Here's how the part is built. I have some questions about the finished solid (model axes, mm). A direction names the side the tool comes from. Coordinates: 2 decimals unless noted, no trailing zeros. Write each loop counter-clockwise with the first axis right and the second up, starting at its lowest first coordinate (ties: lowest second). Pieces come first, ordered by that corner, then holes.
Item 1: If we section it at C-C (x = 7): Count the separate pieces of the cut face and the enclosed holes in it, then the cut area to 3 significant figures.
Item 2: For faces 4 (the face through (-27.75, 4.08, 36.34)), 5 (the face through (-28.414, 5.42, 32.282)), 6 (the face through (23, 5, 31)), 7 (the face through (0, 30, 1)), 8 (the face through (20, 13, 36)), which set-ups out of +Z, -Z, +X, -X, +Y, -Y let a thin tool reach every point of the face, with its end or its side?
Item 3: I'm going to push flat-ended pins straight in: pin 1 Ø0.8 at (x, z) = (-26, 32.5) entering from -Y; pin 2 Ø2 at (y, z) = (9.5, -29.5) entering from -X; pin 3 Ø4.5 at (x, y) = (-24.5, 4.5) entering from -Z; pin 4 Ø1.7 at (x, y) = (27, 4) entering from -Z. Where does each tip first touch, or does it pass through?
Item 4: If I drill on line 1 (Y direction, x = 26, z = 35); line 2 (X direction, y = 4, z = 29); line 3 (X direction, y = 8.1, z = 29), over which ranges is the centre line in solid material (lowest first)?
Item 5: If we section it at D-D (x = 16.5): Please give me the cut outline in (y, z).
Item 6: If we section it at A-A (z = 29): Please give me the cut outline in (x, y).
Item 7: If we section it at B-B (y = 20): Please give me the cut outline in (x, z), then the cut area to 3 significant figures.
Item 8: We'd pull the mould along Z, two halves only. Please class faces 1 (the face through (30, 29, 35)), 2 (the face through (9, 5.9, 31)), 3 (the face through (0, 13, -39)): +Z half, -Z half, draft (parallel to the pull), parting line (faces both ways), or undercut.
from build123d import *

# Parameters (mm, degrees)
SKETCH_1_W                 = 44
SKETCH_1_H                 = 78
EXTRUDE_1_DEPTH            = 33
SHELL_1_T                  = -3
SHELL_1_THICKNESS_2_FACE_W = 75
SHELL_1_THICKNESS_2_FACE_H = 38
SHELL_1_THICKNESS_2_DEPTH  = 7
SKETCH_3_R                 = 3.6
CUT_EXTRUDE_1_DEPTH        = 4.1
CUT_EXTRUDE_2_REACH        = 52.339
SKETCH_4_R                 = 2.25
SKETCH_5_W                 = 3
SKETCH_5_H                 = 3
CUT_EXTRUDE_3_DEPTH        = 6
SKETCH_6_W                 = 8
SKETCH_6_H                 = 8
SKETCH_6_R                 = 1.75
EXTRUDE_2_DEPTH            = 8
CUT_EXTRUDE_4_DEPTH        = 2.6
CUT_EXTRUDE_5_REACH        = 89.258
SKETCH_8_R                 = 5
CUT_EXTRUDE_6_REACH        = 61.245
SKETCH_9_R                 = 3.6


with BuildPart() as part:
    # 草圖1 → 填料-伸長1 (new body)
    with BuildSketch(Plane(origin=(0, 0, 0), x_dir=(1, 0, 0), z_dir=(0, 1, 0))):
        Rectangle(SKETCH_1_W, SKETCH_1_H)
    extrude(amount=EXTRUDE_1_DEPTH)

    # 薄殼1
    shell_1_openings = [part.faces().sort_by_distance(p)[0] for p in [
        (0, 16.5, 39),
    ]]
    offset(amount=SHELL_1_T, openings=shell_1_openings, kind=Kind.INTERSECTION)

    # 薄殼1 thickness 2 face (on inner face of the shell) → 薄殼1 thickness 2 (add)
    with BuildSketch(Plane(origin=(0, 3, 1.5), x_dir=(0, 0, -1), z_dir=(0, -1, 0))):
        Rectangle(SHELL_1_THICKNESS_2_FACE_W, SHELL_1_THICKNESS_2_FACE_H)
    extrude(amount=-SHELL_1_THICKNESS_2_DEPTH)

    # 草圖3 → 除料-伸長1 (cut)
    with BuildSketch(Plane(origin=(0, 10, 0), x_dir=(1, 0, 0), z_dir=(0, 1, 0))):
        with Locations(Location((7, 7, 0), (0, 0, 270))):
            Circle(SKETCH_3_R)
        with Locations(Location((7, -29, 0), (0, 0, 270))):
            Circle(SKETCH_3_R)
    extrude(amount=-CUT_EXTRUDE_1_DEPTH, mode=Mode.SUBTRACT)

    # 草圖4 → 除料-伸長2 (cut, up to next)
    with BuildSketch(Plane(origin=(0, 10, 0), x_dir=(1, 0, 0), z_dir=(0, 1, 0)), mode=Mode.PRIVATE) as cut_extrude_2_sk1:
        with Locations(Location((7, 7, 0), (0, 0, 270))):
            Circle(SKETCH_4_R)
    cut_extrude_2_tool1 = extrude(cut_extrude_2_sk1.sketch, amount=-CUT_EXTRUDE_2_REACH, mode=Mode.PRIVATE) & part.part
    # 草圖4 → 除料-伸長2 (cut, up to next)
    with BuildSketch(Plane(origin=(0, 10, 0), x_dir=(1, 0, 0), z_dir=(0, 1, 0)), mode=Mode.PRIVATE) as cut_extrude_2_sk2:
        with Locations(Location((7, -29, 0), (0, 0, 270))):
            Circle(SKETCH_4_R)
    cut_extrude_2_tool2 = extrude(cut_extrude_2_sk2.sketch, amount=-CUT_EXTRUDE_2_REACH, mode=Mode.PRIVATE) & part.part
    add(cut_extrude_2_tool1.solids().sort_by_distance((7, 10, -7))[0], mode=Mode.SUBTRACT)
    add(cut_extrude_2_tool2.solids().sort_by_distance((7, 10, 29))[0], mode=Mode.SUBTRACT)

    # 草圖5 → 除料-伸長3 (cut)
    with BuildSketch(Plane.XY.offset(39)):
        with Locations((20.5, 11.5)):
            Rectangle(SKETCH_5_W, SKETCH_5_H)
    extrude(amount=-CUT_EXTRUDE_3_DEPTH, mode=Mode.SUBTRACT)

    # 草圖6 → 填料-伸長2 (add)
    with BuildSketch(Plane.XY.offset(39)):
        with Locations((-26, 29)):
            Rectangle(SKETCH_6_W, SKETCH_6_H)
        with Locations((-26, 29)):
            Circle(SKETCH_6_R, mode=Mode.SUBTRACT)
        with Locations((-26, 4)):
            Rectangle(SKETCH_6_W, SKETCH_6_H)
        with Locations((-26, 4)):
            Circle(SKETCH_6_R, mode=Mode.SUBTRACT)
        with Locations((26, 4)):
            Rectangle(SKETCH_6_W, SKETCH_6_H)
        with Locations(Location((26, 4, 0), (0, 0, 180))):
            Circle(SKETCH_6_R, mode=Mode.SUBTRACT)
        with Locations((26, 29)):
            Rectangle(SKETCH_6_W, SKETCH_6_H)
        with Locations(Location((26, 29, 0), (0, 0, 180))):
            Circle(SKETCH_6_R, mode=Mode.SUBTRACT)
    extrude(amount=-EXTRUDE_2_DEPTH)

    # 草圖7 → 除料-伸長4 (cut)
    with BuildSketch(Plane(origin=(0, 0, 31), x_dir=(-1, 0, 0), z_dir=(0, 0, -1))):
        Polygon((27.616580754, 6.8), (29.233161507, 4), (27.616580754, 1.2), (24.383419246, 1.2), (22.766838493, 4), (24.383419246, 6.8), align=None)
        Polygon((-22.766838493, 29), (-24.383419246, 31.8), (-27.616580754, 31.8), (-29.233161507, 29), (-27.616580754, 26.2), (-24.383419246, 26.2), align=None)
        Polygon((-29.233161507, 4), (-27.616580754, 1.2), (-24.383419246, 1.2), (-22.766838493, 4), (-24.383419246, 6.8), (-27.616580754, 6.8), align=None)
        Polygon((24.383419246, 26.2), (22.766838493, 29), (24.383419246, 31.8), (27.616580754, 31.8), (29.233161507, 29), (27.616580754, 26.2), align=None)
    extrude(amount=-CUT_EXTRUDE_4_DEPTH, mode=Mode.SUBTRACT)

    # 草圖8 → 除料-伸長5 (cut, up to next)
    with BuildSketch(Plane.XY.offset(-36), mode=Mode.PRIVATE) as cut_extrude_5_sk1:
        with Locations((0, 20)):
            Circle(SKETCH_8_R)
    cut_extrude_5_tool1 = extrude(cut_extrude_5_sk1.sketch, amount=-CUT_EXTRUDE_5_REACH, mode=Mode.PRIVATE) & part.part
    add(cut_extrude_5_tool1.solids().sort_by_distance((0, 20, -36))[0], mode=Mode.SUBTRACT)

    # 草圖9 → 除料-伸長6 (cut, up to next)
    with BuildSketch(Plane(origin=(0, 33, 0), x_dir=(1, 0, 0), z_dir=(0, 1, 0)), mode=Mode.PRIVATE) as cut_extrude_6_sk1:
        with Locations(Location((7, 7, 0), (0, 0, 270))):
            Circle(SKETCH_9_R)
    cut_extrude_6_tool1 = extrude(cut_extrude_6_sk1.sketch, amount=-CUT_EXTRUDE_6_REACH, mode=Mode.PRIVATE) & part.part
    # 草圖9 → 除料-伸長6 (cut, up to next)
    with BuildSketch(Plane(origin=(0, 33, 0), x_dir=(1, 0, 0), z_dir=(0, 1, 0)), mode=Mode.PRIVATE) as cut_extrude_6_sk2:
        with Locations(Location((7, -29, 0), (0, 0, 270))):
            Circle(SKETCH_9_R)
    cut_extrude_6_tool2 = extrude(cut_extrude_6_sk2.sketch, amount=-CUT_EXTRUDE_6_REACH, mode=Mode.PRIVATE) & part.part
    add(cut_extrude_6_tool1.solids().sort_by_distance((7, 33, -7))[0], mode=Mode.SUBTRACT)
    add(cut_extrude_6_tool2.solids().sort_by_distance((7, 33, 29))[0], mode=Mode.SUBTRACT)


solid = part.part
Answer list:
1. separate pieces: 5
1. enclosed holes: 0
1. area: 919 mm2
2. face 4: +Z, -Z
2. face 5: -Z
2. face 6: -Z, +X, +Y, -Y
2. face 7: +Z
2. face 8: +Z, +X
3. pin 1: stops at y = 0
3. pin 2: stops at x = -22
3. pin 3: stops at z = 31
3. pin 4: stops at z = 33.6
4. line 1: y = 0 to 2.25, 5.75 to 8, 25 to 27.25, 30.75 to 33
4. line 2: x = -22 to 4.75, 9.25 to 22
4. line 3: x = -22 to 3.4, 10.6 to 22
5. outline: (0, -39) - (33, -39) - (33, 39) - (30, 39) - (30, -36) - (10, -36) - (10, 39) - (0, 39) - close
6. outline: (-22, 0) - (4.75, 0) - (4.75, 5.9) - (3.4, 5.9) - (3.4, 10) - (-19, 10) - (-19, 30) - (3.4, 30) - (3.4, 33) - (-22, 33) - close; (9.25, 0) - (22, 0) - (22, 33) - (10.6, 33) - (10.6, 30) - (19, 30) - (19, 10) - (10.6, 10) - (10.6, 5.9) - (9.25, 5.9) - close
7. outline: (-22, -39) - (-5, -39) - (-5, -36) - (-19, -36) - (-19, 39) - (-22, 39) - close; (5, -39) - (22, -39) - (22, 39) - (19, 39) - (19, -36) - (5, -36) - close
7. area: 552 mm2
8. face 1: draft
8. face 2: undercut
8. face 3: -Z half
